The model under review builds one solid part; all positions refer to its coordinate system, in mm. Coordinates: 2 decimals unless noted, no trailing zeros. Loops run counter-clockwise (first coordinate to the right, second up) from the corner with the lowest first, then second, coordinate; pieces in that order, holes last. Notation, with made-up numbers: (13, -18) - (59, -18) arc R37 cw to (59, 21) - close; hole circle Ø3 at (-20.5, -0.75). An arc over 180 degrees is marked (long way). Use a Markdown table: item, result. Add a question column.
1) To check wall thickness, follow L1, parallel to Z at x = 3, y = -131; L2, parallel to X at y = -25, z = 2.25. State the ranges of each line that lie inside material, in increasing order. Write a range as [from, to].
2) Clearance check with flat-ended pins moving along their axes: pin 1 (1 mm diameter, centred on x = 3, y = -367, fed in from +Z); pin 2 (3 mm diameter, centred on y = -181, z = 2.5, fed in from +X). State where each tip first meets the part, or that it passes through.
3) Add section B-B, the plane z = 3. Give the boundary of the cut face in (x, y).
4) Add section A-A, the plane y = -193.5. Give the boundary of the cut face in (x, z), and give its area (3 significant figures).
```python
from build123d import *

# Parameters (mm, degrees)
F0_W     = 0.882425
F0_H     = 5.536785
F0_W_2   = 5.467575
F0_H_2   = 0.813215
F1_DEPTH = 463.55
F2_R     = 1.264941
F3_DEPTH = 25.4
F4_R     = 1.275366
F5_DEPTH = 25.4


with BuildPart() as f1:
    # F0 (on Front) → F1 (new body)
    with BuildSketch(Plane.XZ):
        with Locations((0.441213, 3.581607)):
            Rectangle(F0_W, F0_H)
        with Locations((3.616212, 0.406607)):
            Rectangle(F0_W_2, F0_H_2)
        with Locations((0.441213, 0.406607)):
            Rectangle(F0_W, F0_H_2)
    extrude(amount=F1_DEPTH)

    # F2 (on face) → F3 (cut)
    with BuildSketch(Plane.XY.offset(0.813215)):
        with Locations((3.616212, -2.749367)):
            Circle(F2_R)
    extrude(amount=-F3_DEPTH, mode=Mode.SUBTRACT)

    # F4 (on face) → F5 (cut)
    with BuildSketch(Plane.XY.offset(0.813215)):
        with Locations((3.616212, -460.805912)):
            Circle(F4_R)
    extrude(amount=-F5_DEPTH, mode=Mode.SUBTRACT)


solid = f1.part
```
From the geometry:
| question | item | result |
|---|---|---|
| 1 | L1 | z = [0, 0.81] |
| 1 | L2 | x = [0, 0.88] |
| 2 | pin 1 | stops at z = 0.81 |
| 2 | pin 2 | stops at x = 0.88 |
| 3 | outline | (0, -463.55) - (0.88, -463.55) - (0.88, 0) - (0, 0) - close |
| 4 | outline | (0, 0) - (6.35, 0) - (6.35, 0.81) - (0.88, 0.81) - (0.88, 6.35) - (0, 6.35) - close |
| 4 | area | 10.0 mm^2 |
